Design review of the part built by this model. Coordinates are the model's own, in mm. A direction names the side the tool comes from. Coordinates: 2 decimals unless noted, no trailing zeros. Loops run counter-clockwise (first coordinate to the right, second up) from the corner with the lowest first, then second, coordinate; pieces in that order, holes last. Notation, with made-up numbers: (15.25, -16) -> (31.25, -16) arc R30 cw to (31.25, 11) -> close; hole circle Ø10 at (50, -10.75). An arc over 180 degrees is marked (long way). Answer in a Markdown table with one row per item.
```python
from build123d import *

# Parameters (mm, degrees)
SKETCH2_R           = 3.75
BOSS_EXTRUDE1_DEPTH = 3.75
SKETCH3_R           = 1.875
BOSS_EXTRUDE2_DEPTH = 1.25
SKETCH4_R           = 5.625
CUT_EXTRUDE1_DEPTH  = 0.75
SKETCH5_R           = 5.5
SKETCH5_R_2         = 2.875
BOSS_EXTRUDE3_DEPTH = 0.75
SKETCH7_R           = 1.875
BOSS_EXTRUDE4_DEPTH = 1.25
SKETCH8_R           = 6.25
CUT_EXTRUDE2_DEPTH  = 25


with BuildPart() as part:
    # Sketch1 → Revolve1 (revolve)
    with BuildSketch(Plane.XY):
        Polygon((-22.785, 0), (22.785, 0), (22.785, 18.15), (20.285, 18.15), (20.285, 25), (4.715, 25), (4.715, 40.65), (20.965, 40.65), (20.965, 45), (30.965, 45), (30.965, 50), (33.465, 50), (33.465, 52.5), (27.965, 52.5), (27.965, 46.9), (-34.035, 46.9), (-34.035, 42.5), (-26.535, 42.5), (-26.535, 40.65), (-14.535, 40.65), (-14.535, 22.5), (-19.035, 22.5), (-19.035, 16.25), (-22.785, 16.25), align=None)
    revolve(axis=Axis((-22.785, 0, 0), (1, 0, 0)))

    # Sketch2 → Boss-Extrude1 (add)
    with BuildSketch(Plane(origin=(4.715, 0, 0), x_dir=(0, 0, -1), z_dir=(1, 0, 0))):
        with Locations((0, 31.25)):
            Circle(SKETCH2_R)
        with Locations((15.625, 27.063293868)):
            Circle(SKETCH2_R)
        with Locations((27.063293868, 15.625)):
            Circle(SKETCH2_R)
        with Locations((31.25, 0)):
            Circle(SKETCH2_R)
        with Locations((27.063293868, -15.625)):
            Circle(SKETCH2_R)
        with Locations((15.625, -27.063293868)):
            Circle(SKETCH2_R)
        with Locations((0, -31.25)):
            Circle(SKETCH2_R)
        with Locations((-15.625, -27.063293868)):
            Circle(SKETCH2_R)
        with Locations((-27.063293868, -15.625)):
            Circle(SKETCH2_R)
        with Locations((-31.25, 0)):
            Circle(SKETCH2_R)
        with Locations((-27.063293868, 15.625)):
            Circle(SKETCH2_R)
        with Locations((-15.625, 27.063293868)):
            Circle(SKETCH2_R)
    extrude(amount=BOSS_EXTRUDE1_DEPTH)

    # Sketch3 → Boss-Extrude2 (add)
    with BuildSketch(Plane(origin=(20.285, 0, 0), x_dir=(0, 0, -1), z_dir=(1, 0, 0))):
        with Locations((0, 21.25)):
            Circle(SKETCH3_R)
        with Locations((10.625, 18.40303983)):
            Circle(SKETCH3_R)
        with Locations((18.40303983, 10.625)):
            Circle(SKETCH3_R)
        with Locations((21.25, 0)):
            Circle(SKETCH3_R)
        with Locations((18.40303983, -10.625)):
            Circle(SKETCH3_R)
        with Locations((10.625, -18.40303983)):
            Circle(SKETCH3_R)
        with Locations((0, -21.25)):
            Circle(SKETCH3_R)
        with Locations((-10.625, -18.40303983)):
            Circle(SKETCH3_R)
        with Locations((-18.40303983, -10.625)):
            Circle(SKETCH3_R)
        with Locations((-21.25, 0)):
            Circle(SKETCH3_R)
        with Locations((-18.40303983, 10.625)):
            Circle(SKETCH3_R)
        with Locations((-10.625, 18.40303983)):
            Circle(SKETCH3_R)
    extrude(amount=BOSS_EXTRUDE2_DEPTH)

    # Sketch4 → Cut-Extrude1 (cut)
    with BuildSketch(Plane(origin=(22.785, 0, 0), x_dir=(0, 0, -1), z_dir=(1, 0, 0))):
        Circle(SKETCH4_R)
    extrude(amount=-CUT_EXTRUDE1_DEPTH, mode=Mode.SUBTRACT)

    # Sketch5 → Boss-Extrude3 (add)
    with BuildSketch(Plane(origin=(22.785, 0, 0), x_dir=(0, 0, -1), z_dir=(1, 0, 0))):
        with Locations((0, 11.875)):
            Circle(SKETCH5_R)
        with Locations((0, 11.875)):
            Circle(SKETCH5_R_2, mode=Mode.SUBTRACT)
        with Locations((10.28405167, -5.9375)):
            Circle(SKETCH5_R)
        with Locations((10.28405167, -5.9375)):
            Circle(SKETCH5_R_2, mode=Mode.SUBTRACT)
        with Locations((-10.28405167, -5.9375)):
            Circle(SKETCH5_R)
        with Locations((-10.28405167, -5.9375)):
            Circle(SKETCH5_R_2, mode=Mode.SUBTRACT)
    extrude(amount=BOSS_EXTRUDE3_DEPTH)

    # Sketch7 → Boss-Extrude4 (add)
    with BuildSketch(Plane.ZY.offset(19.035)):
        with Locations((0, 19.05)):
            Circle(SKETCH7_R)
        with Locations((9.525, 16.497783942)):
            Circle(SKETCH7_R)
        with Locations((16.497783942, 9.525)):
            Circle(SKETCH7_R)
        with Locations((19.05, 0)):
            Circle(SKETCH7_R)
        with Locations((16.497783942, -9.525)):
            Circle(SKETCH7_R)
        with Locations((9.525, -16.497783942)):
            Circle(SKETCH7_R)
        with Locations((0, -19.05)):
            Circle(SKETCH7_R)
        with Locations((-9.525, -16.497783942)):
            Circle(SKETCH7_R)
        with Locations((-16.497783942, -9.525)):
            Circle(SKETCH7_R)
        with Locations((-19.05, 0)):
            Circle(SKETCH7_R)
        with Locations((-16.497783942, 9.525)):
            Circle(SKETCH7_R)
        with Locations((-9.525, 16.497783942)):
            Circle(SKETCH7_R)
    extrude(amount=BOSS_EXTRUDE4_DEPTH)

    # Sketch8 → Cut-Extrude2 (cut)
    with BuildSketch(Plane.ZY.offset(22.785)):
        Circle(SKETCH8_R)
    extrude(amount=-CUT_EXTRUDE2_DEPTH, mode=Mode.SUBTRACT)


solid = part.part
```
(1) Tool access review of faces 1 (the flat face through (-20.285, 10, 16)), 2 (the flat face through (21.535, -11, 18)): name each direction out of +Z, -Z, +X, -X, +Y, -Y from which nothing blocks a thin tool from reaching the whole face with its end or side.
Evaluation:
| item | result |
|---|---|
| face 1 | -X |
| face 2 | +X |
(2) For pin 1 (1.1 mm diameter, centred on y = -17, z = -9, fed in from -X) (3 decimals); pin 2 (2 mm diameter, centred on x = 20, y = 38.5, fed in from +Z); pin 3 (1.5 mm diameter, centred on x = -13, y = -23.5, fed in from +Z), all flat-tipped, find the tip position at first contact; note any pin that passes through.
Evaluation:
| item | result |
|---|---|
| pin 1 | stops at x = -20.285 |
| pin 2 | stops at z = 28.17 |
| pin 3 | stops at z = 41.01 |
(3) Take a section at A-A on x = 16.5. Give the boundary of the cut face in (y, z).
Evaluation:
| item | result |
|---|---|
| outline | circle Ø93.8 at (0, 0); circle Ø50 at (0, 0); hole circle Ø81.3 at (0, 0) |
(4) To check wall thickness, follow probe 1 along Z at (x, y) = (22, 0); probe 2 along Y at (x, z) = (18, 10); probe 3 along Z at (x, y) = (24.5, 0). State the ranges of each line that lie inside material, in increasing order.
Evaluation:
| item | result |
|---|---|
| probe 1 | z = -46.9 to -45, -18.15 to 18.15, 45 to 46.9 |
| probe 2 | y = -45.82 to -39.4, -22.91 to 22.91, 39.4 to 45.82 |
| probe 3 | z = -46.9 to -45, 45 to 46.9 |
(5) Take a section at C-C on x = -5. Give the boundary of the cut face in (y, z).
Evaluation:
| item | result |
|---|---|
| outline | circle Ø93.8 at (0, 0); hole circle Ø12.5 at (0, 0) |
(6) Take a section at B-B on z = 39. Give the boundary of the cut face in (x, y) (3 decimals), and give its area (3 significant figures).
Evaluation:
| item | result |
|---|---|
| outline | (-34.035, -26.05) -> (27.965, -26.05) -> (27.965, -35.146) -> (33.465, -35.146) -> (33.465, -31.289) -> (30.965, -31.289) -> (30.965, -22.45) -> (20.965, -22.45) -> (20.965, -11.464) -> (4.715, -11.464) -> (4.715, 11.464) -> (20.965, 11.464) -> (20.965, 22.45) -> (30.965, 22.45) -> (30.965, 31.289) -> (33.465, 31.289) -> (33.465, 35.146) -> (27.965, 35.146) -> (27.965, 26.05) -> (-34.035, 26.05) -> (-34.035, 16.889) -> (-26.535, 16.889) -> (-26.535, 11.464) -> (-14.535, 11.464) -> (-14.535, -11.464) -> (-26.535, -11.464) -> (-26.535, -16.889) -> (-34.035, -16.889) -> close |
| area | 2,110 mm² |
